```python
from build123d import *

# Parameters (mm, degrees)
BOSS_EXTRUDE1_DEPTH = 3.15
SKETCH3_R           = 2.45
BOSS_EXTRUDE2_DEPTH = 1.95
SHELL1_T            = -1.5


with BuildPart() as part:
    # Sketch2 → Boss-Extrude1 (new body)
    with BuildSketch(Plane(origin=(0, 0, 0), x_dir=(1, 0, 0), z_dir=(0, 1, 0))):
        Polygon((0, 0), (0, -7.925), (-7.925, -7.925), (-7.925, 7.925), (7.925, 7.925), (7.925, 0), align=None)
    extrude(amount=-BOSS_EXTRUDE1_DEPTH)

    # Sketch3 → Boss-Extrude2 (add)
    with BuildSketch(Plane(origin=(0, 0, 0), x_dir=(1, 0, 0), z_dir=(0, 1, 0))):
        with Locations(Location((-3.9625, 3.9625, 0), (0, 0, 270))):
            Circle(SKETCH3_R)
        with Locations(Location((3.9625, 3.9625, 0), (0, 0, 270))):
            Circle(SKETCH3_R)
        with Locations(Location((-3.9625, -3.9625, 0), (0, 0, 270))):
            Circle(SKETCH3_R)
    extrude(amount=BOSS_EXTRUDE2_DEPTH)

    # Shell1
    shell1_openings = [part.faces().sort_by_distance(p)[0] for p in [
        (-1.320833333, -3.15, -1.320833333),
    ]]
    offset(amount=SHELL1_T, openings=shell1_openings, kind=Kind.INTERSECTION)


solid = part.part
```
Work out the finished part from the listing and answer in its coordinate system (mm). A direction names the side the tool comes from. Give positions to 0.01 mm unless a question says otherwise; leave off trailing zeros. Loops run counter-clockwise (first coordinate to the right, second up) from the corner with the lowest first, then second, coordinate; pieces in that order, holes last. Notation, with made-up numbers: (80, 60.5) -> (108, 60.5) arc R19 cw to (108, 86.5) -> close; hole circle Ø1 at (82.25, 38). An arc over 180 degrees is marked (long way). Put each result on its own line as item: value. Start each with the question number.
Item 1: The part is cut by section B-B (z = 1). Give the vertices of the cut face in (x, y) (3 decimals).
Item 2: The mould has two halves that part along X. Classify faces 5 (the face through (-7.925, -2, 0)), 6 (the face through (4, 1.95, -4)), 7 (the face through (6.425, -2, -4)): released by +X, released by -X, zero draft, split by the parting line, or undercut.
Item 3: The part is cut by section D-D (y = 0.2). Give the vertices of the cut face in (x, z).
Item 4: Each of these flat-tipped pins is pushed along its axis until it touches: P1, Ø1.3, axis at x = 3, y = -2.5, coming from the +Z side; P2, Ø1.6, axis at y = -1.5, z = 4.5, coming from the +X side; P3, Ø1.5, axis at x = -3.96, z = 3.96, coming from the -Y side. Where does it stop, or does it pass through?
Item 5: Find the intervals of material crossed by L1, parallel to X at y = -2.35, z = -5.5 (3 decimals); L2, parallel to X at y = -2.2, z = 1 (3 decimals), in increasing order. Write a range as [from, to].
Item 6: The part is cut by section C-C (x = 0.75). Give the vertices of the cut face in (y, z) (3 decimals).
Item 7: The part is cut by section A-A (y = -2.3). Give the vertices of the cut face in (x, z) (3 decimals), then the cut area to 3 significant figures.
Item 8: Which of the six approach directions +Z, -Z, +X, -X, +Y, -Y give full straight-line access (tool end or side, diameter ignored) to faces 1 (the face through (4, 0.45, -4)), 2 (the face through (-2, 0, -2)), 3 (the face through (-4, 1.95, 4)), 4 (the face through (0, -2, 4))?
Answers below:
1. outline: (-7.925, -3.15) -> (-6.425, -3.15) -> (-6.425, -1.5) -> (-1.5, -1.5) -> (-1.5, -3.15) -> (0, -3.15) -> (0, 0) -> (-7.925, 0) -> close
2. face 5: released by -X
2. face 6: zero draft
2. face 7: undercut
3. outline: circle Ø4.9 at (-3.96, -3.96); circle Ø4.9 at (-3.96, 3.96); circle Ø4.9 at (3.96, -3.96); hole circle Ø1.9 at (-3.96, -3.96); hole circle Ø1.9 at (-3.96, 3.96); hole circle Ø1.9 at (3.96, -3.96)
4. P1: z = 0
4. P2: x = 0
4. P3: y = 0.45
5. L1: [-7.925, -6.425], [6.425, 7.925]
5. L2: [-7.925, -6.425], [-1.5, 0]
6. outline: (-3.15, -7.925) -> (0, -7.925) -> (0, 0) -> (-3.15, 0) -> (-3.15, -1.5) -> (-1.5, -1.5) -> (-1.5, -6.425) -> (-3.15, -6.425) -> close
7. outline: (-7.925, -7.925) -> (7.925, -7.925) -> (7.925, 0) -> (0, 0) -> (0, 7.925) -> (-7.925, 7.925) -> close; hole (-6.425, -6.425) -> (6.425, -6.425) -> (6.425, -1.5) -> (-1.5, -1.5) -> (-1.5, 6.425) -> (-6.425, 6.425) -> close
7. area: 86.1 mm2
8. face 1: -Y
8. face 2: +Y
8. face 3: +Z, -Z, +X, -X, +Y
8. face 4: +Z, +X, +Y, -Y
